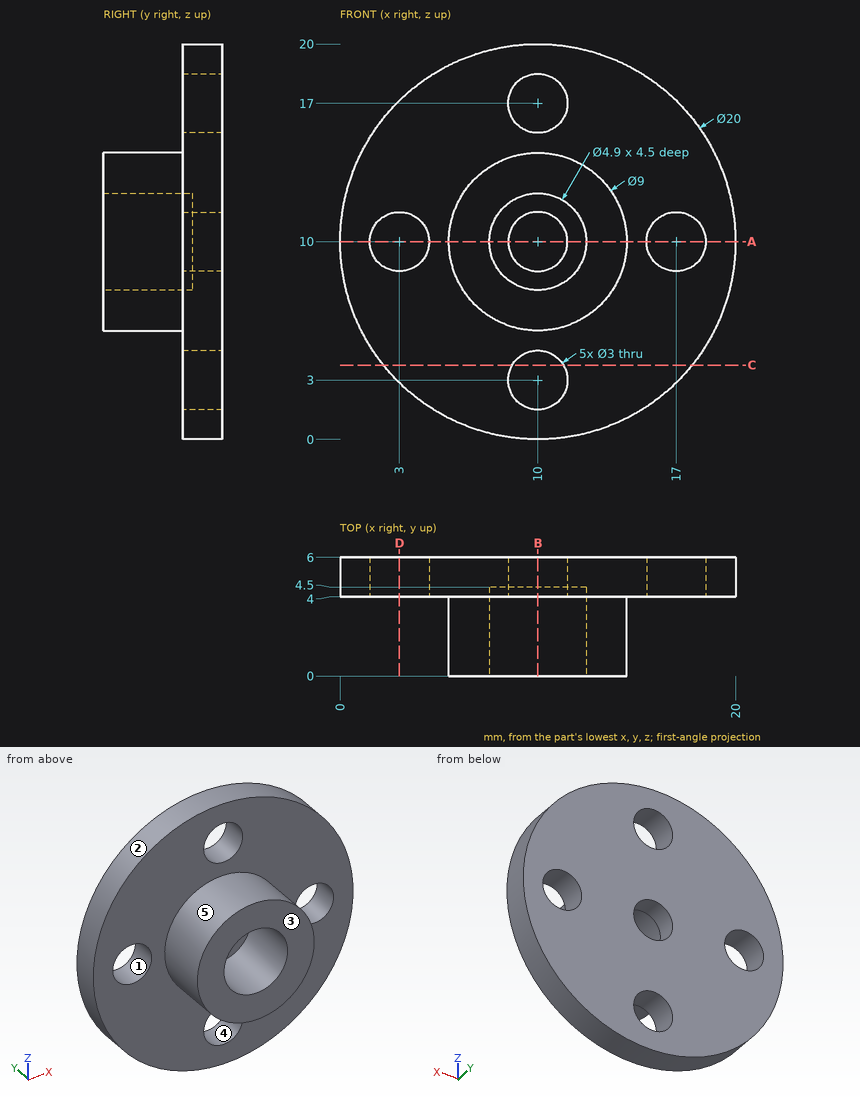
Geometry check sheet. Reference: drawing and pictorial views, mm from the part's lowest x, y, z. A direction names the side the tool comes from. Coordinates: 2 decimals unless noted, no trailing zeros. Loops run counter-clockwise (first coordinate to the right, second up) from the corner with the lowest first, then second, coordinate; pieces in that order, holes last.
1) Sectioned sample at D-D (x = 3). Record the boundary of the cut face in (y, z).
2) Gauge pin test, flat ends, axial feed: pin 1 (4 mm diameter, centred on x = 3, z = 10, fed in from -Y); pin 2 (1.5 mm diameter, centred on y = 5.5, z = 5, fed in from +X); pin 3 (2.5 mm diameter, centred on x = 10, z = 10.5, fed in from -Y). Record the tip position at first contact, or that the pin passes through.
3) Sectioned sample at C-C (z = 3.75). Record the boundary of the cut face in (x, y), and give its area (3 significant figures).
4) Release check for a two-part mould opening along Z. For the marked faces 1, 2 and 3 record: released by +Z, released by -Z, zero draft, split by the parting line, or undercut.
5) Sectioned sample at A-A (z = 10). Record the boundary of the cut face in (x, y), and give its area (4 significant figures).
6) Material ranges on probe 1 along X at (y, z) = (5, 10); probe 2 along Y at (x, z) = (18, 12.75); probe 3 along Z at (x, y) = (10.5, 2.5), recorded low to high.
7) Sectioned sample at B-B (x = 10). Record the boundary of the cut face in (y, z).
8) Access from +Z, -Z, +X, -X, +Y, -Y to the whole of each face (thin tool, end or side, straight path). Record for the marked faces 4 and 5.
Check sheet entries:
1. outline: (4, 2.86) - (6, 2.86) - (6, 8.5) - (4, 8.5) - close; (4, 11.5) - (6, 11.5) - (6, 17.14) - (4, 17.14) - close
2. pin 1: stops at y = 4
2. pin 2: stops at x = 19.05
2. pin 3: stops at y = 4.5
3. outline: (2.19, 4) - (8.7, 4) - (8.7, 6) - (2.19, 6) - close; (11.3, 4) - (17.81, 4) - (17.81, 6) - (11.3, 6) - close
3. area: 26.0 mm2
4. face 1: undercut
4. face 2: split by the parting line
4. face 3: zero draft
5. outline: (0, 4) - (1.5, 4) - (1.5, 6) - (0, 6) - close; (4.5, 4) - (5.5, 4) - (5.5, 0) - (7.55, 0) - (7.55, 4.5) - (8.5, 4.5) - (8.5, 6) - (4.5, 6) - close; (11.5, 4.5) - (12.45, 4.5) - (12.45, 0) - (14.5, 0) - (14.5, 4) - (15.5, 4) - (15.5, 6) - (11.5, 6) - close; (18.5, 4) - (20, 4) - (20, 6) - (18.5, 6) - close
5. area: 37.45 mm2
6. probe 1: x = 0 to 1.5, 4.5 to 8.5, 11.5 to 15.5, 18.5 to 20
6. probe 2: y = 4 to 6
6. probe 3: z = 5.53 to 7.6, 12.4 to 14.47
7. outline: (0, 5.5) - (4, 5.5) - (4, 4.5) - (6, 4.5) - (6, 8.5) - (4.5, 8.5) - (4.5, 7.55) - (0, 7.55) - close; (0, 12.45) - (4.5, 12.45) - (4.5, 11.5) - (6, 11.5) - (6, 15.5) - (4, 15.5) - (4, 14.5) - (0, 14.5) - close; (4, 0) - (6, 0) - (6, 1.5) - (4, 1.5) - close; (4, 18.5) - (6, 18.5) - (6, 20) - (4, 20) - close
8. face 4: +Y, -Y
8. face 5: -Y
